from build123d import *

# Parameters (mm, degrees)
F0_R     = 1.5875
F1_DEPTH = 3.048


with BuildPart() as f1:
    # F0 (on Front) → F1 (new body)
    with BuildSketch(Plane.XZ):
        with BuildLine():
            Line((0, 112.7125), (0, 104.775))
            ThreePointArc((0, 104.775), (6.7351920908, 107.5648079092), (9.525, 114.3))
            Line((9.525, 114.3), (1.5875, 114.3))
            ThreePointArc((1.5875, 114.3), (1.1225320151, 113.1774679849), (0, 112.7125))
        make_face()
        with BuildLine():
            Line((-1.5875, 114.3), (-9.525, 114.3))
            ThreePointArc((-9.525, 114.3), (-6.7351920908, 107.5648079092), (0, 104.775))
            Line((0, 104.775), (0, 112.7125))
            ThreePointArc((0, 112.7125), (-1.1225320151, 113.1774679849), (-1.5875, 114.3))
        make_face()
        with BuildLine():
            ThreePointArc((9.525, 114.3), (0, 123.825), (-9.525, 114.3))
            Line((-9.525, 114.3), (-1.5875, 114.3))
            ThreePointArc((-1.5875, 114.3), (0, 115.8875), (1.5875, 114.3))
            Line((1.5875, 114.3), (9.525, 114.3))
        make_face()
        with BuildLine():
            Line((0, 104.775), (0, 79.375))
            ThreePointArc((0, 79.375), (10.0640474958, 75.7772380038), (15.5664511985, 66.6146784884))
            Line((15.5664511985, 66.6146784884), (9.5992867411, 114.3))
            Line((9.5992867411, 114.3), (9.525, 114.3))
            ThreePointArc((9.525, 114.3), (6.7351920908, 107.5648079092), (0, 104.775))
        make_face()
        with BuildLine():
            Line((-9.525, 114.3), (-15.7474569047, 65.5082893304))
            ThreePointArc((-15.7474569047, 65.5082893304), (-10.4912828548, 75.4142187767), (0, 79.375))
            Line((0, 79.375), (0, 104.775))
            ThreePointArc((0, 104.775), (-6.7351920908, 107.5648079092), (-9.525, 114.3))
        make_face()
        with Locations((-4.7625, 100.0252)):
            Circle(F0_R, mode=Mode.SUBTRACT)
        with BuildLine():
            ThreePointArc((-15.7942028036, 61.9003804205), (-10.644756084, 51.722700101), (0, 47.625))
            Line((0, 47.625), (0, 61.9125))
            ThreePointArc((0, 61.9125), (-1.5875, 63.5), (0, 65.0875))
            Line((0, 65.0875), (0, 79.375))
            ThreePointArc((0, 79.375), (-10.4912828548, 75.4142187767), (-15.7474569047, 65.5082893304))
            ThreePointArc((-15.7474569047, 65.5082893304), (-15.873667691, 63.7056672947), (-15.7942028036, 61.9003804205))
        make_face()
        with BuildLine():
            Line((0, 61.9125), (0, 47.625))
            ThreePointArc((0, 47.625), (10.644756084, 51.722700101), (15.7942028036, 61.9003804205))
            ThreePointArc((15.7942028036, 61.9003804205), (15.8547878338, 62.6991705884), (15.875, 63.5))
            ThreePointArc((15.875, 63.5), (15.7976744772, 65.0649620162), (15.5664511985, 66.6146784884))
            ThreePointArc((15.5664511985, 66.6146784884), (10.0640474958, 75.7772380038), (0, 79.375))
            Line((0, 79.375), (0, 65.0875))
            ThreePointArc((0, 65.0875), (1.1225320151, 64.6225320151), (1.5875, 63.5))
            ThreePointArc((1.5875, 63.5), (1.1225320151, 62.3774679849), (0, 61.9125))
        make_face()
        with BuildLine():
            Line((0, 47.625), (0, 9.525))
            ThreePointArc((0, 9.525), (6.7351920908, 6.7351920908), (9.525, 0))
            Line((9.525, 0), (36.5125, 0))
            ThreePointArc((36.5125, 0), (38.8373399243, 5.6126600757), (44.45, 7.9375))
            Line((44.45, 7.9375), (18.9329889534, 8.8488218231))
            ThreePointArc((18.9329889534, 8.8488218231), (13.22446249, 11.5691841219), (11.3070069952, 17.5950458731))
            Line((11.3070069952, 17.5950458731), (15.7942028036, 61.9003804205))
            ThreePointArc((15.7942028036, 61.9003804205), (10.644756084, 51.722700101), (0, 47.625))
        make_face()
        with BuildLine():
            ThreePointArc((-9.525, 0), (-6.7351920908, 6.7351920908), (0, 9.525))
            Line((0, 9.525), (0, 47.625))
            ThreePointArc((0, 47.625), (-10.644756084, 51.722700101), (-15.7942028036, 61.9003804205))
            Line((-15.7942028036, 61.9003804205), (-9.525, 0))
        make_face()
        with BuildLine():
            Line((0, 9.525), (0, 1.5875))
            ThreePointArc((0, 1.5875), (1.1225320151, 1.1225320151), (1.5875, 0))
            Line((1.5875, 0), (9.525, 0))
            ThreePointArc((9.525, 0), (6.7351920908, 6.7351920908), (0, 9.525))
        make_face()
        with BuildLine():
            ThreePointArc((-1.5875, 0), (-1.1225320151, 1.1225320151), (0, 1.5875))
            Line((0, 1.5875), (0, 9.525))
            ThreePointArc((0, 9.525), (-6.7351920908, 6.7351920908), (-9.525, 0))
            Line((-9.525, 0), (-1.5875, 0))
        make_face()
        with BuildLine():
            ThreePointArc((0, -1.5875), (-1.1225320151, -1.1225320151), (-1.5875, 0))
            Line((-1.5875, 0), (-9.525, 0))
            ThreePointArc((-9.525, 0), (-6.7351920908, -6.7351920908), (0, -9.525))
            Line((0, -9.525), (0, -1.5875))
        make_face()
        with BuildLine():
            Line((9.525, 0), (1.5875, 0))
            ThreePointArc((1.5875, 0), (1.1225320151, -1.1225320151), (0, -1.5875))
            Line((0, -1.5875), (0, -9.525))
            Line((0, -9.525), (0.6773435479, -9.500885786))
            ThreePointArc((0.6773435479, -9.500885786), (6.9705567315, -6.4912990883), (9.525, 0))
        make_face()
        with BuildLine():
            Line((36.5125, 0), (9.525, 0))
            ThreePointArc((9.525, 0), (6.9705567315, -6.4912990883), (0.6773435479, -9.500885786))
            Line((0.6773435479, -9.500885786), (44.45, -7.9425285691))
            Line((44.45, -7.9425285691), (44.45, -7.9375))
            ThreePointArc((44.45, -7.9375), (38.8373399243, -5.6126600757), (36.5125, 0))
        make_face()
        with BuildLine():
            Line((42.8625, 0), (36.5125, 0))
            ThreePointArc((36.5125, 0), (38.8373399243, -5.6126600757), (44.45, -7.9375))
            Line((44.45, -7.9375), (44.45, -1.5875))
            ThreePointArc((44.45, -1.5875), (43.3274679849, -1.1225320151), (42.8625, 0))
        make_face()
        with BuildLine():
            ThreePointArc((44.45, 7.9375), (38.8373399243, 5.6126600757), (36.5125, 0))
            Line((36.5125, 0), (42.8625, 0))
            ThreePointArc((42.8625, 0), (44.45, 1.5875), (46.0375, 0))
            ThreePointArc((46.0375, 0), (45.5725320151, -1.1225320151), (44.45, -1.5875))
            Line((44.45, -1.5875), (44.45, -7.9375))
            ThreePointArc((44.45, -7.9375), (50.0626600757, -5.6126600757), (52.3875, 0))
            ThreePointArc((52.3875, 0), (50.0626600757, 5.6126600757), (44.45, 7.9375))
        make_face()
    extrude(amount=F1_DEPTH)


solid = f1.part
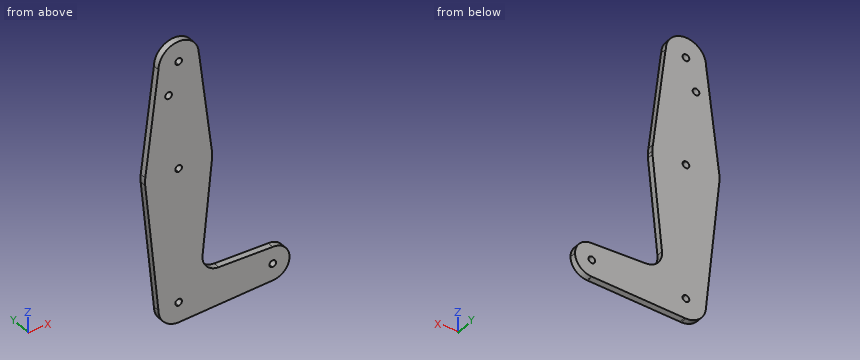
CAD build for the part. Positions are in the model's coordinates, mm. Round coordinates to 2 decimals unless told otherwise and drop trailing zeros. Write each loop counter-clockwise with the first axis right and the second up, starting at its lowest first coordinate (ties: lowest second). Pieces come first, ordered by that corner, then holes. Notation, with made-up numbers: (39.25, 21.5) -> (98.25, 21.5) arc R24 cw to (98.25, 43.5) -> close; hole circle Ø7 at (24, 86.25). An arc over 180 degrees is marked (long way). Answer as a JSON object with one key per item and string values.
(1) Band-saw the part on A-A, the plane y = -1. Count the separate pieces of the cut face and the enclosed holes in it, then the cut area to 3 significant figures.
Reported:
{"separate pieces": "1", "enclosed holes": "5", "area": "3,890 mm^2"}
(2) Probe probe 1 along X at (y, z) = (-0.55, -0.5); probe 2 along X at (y, z) = (-2.85, 104); probe 3 along X at (y, z) = (-2.9, 32). List the from-to ranges inside material, lowest first. Write a range as [from, to].
Reported:
{"probe 1": "x = [-9.51, -1.51], [1.51, 42.94], [45.96, 52.37]", "probe 2": "x = [-10.84, 10.89]", "probe 3": "x = [-12.77, 12.77]"}
(3) Band-saw the part on B-B, the plane z = 49. List the corners of the cut face in (x, y).
Reported:
{"outline": "(-14.49, -3.05) -> (14.49, -3.05) -> (14.49, 0) -> (-14.49, 0) -> close"}
(4) Pin check, flat tips, straight feed: P1, Ø1, axis at x = 3.5, y = -2, coming from the -Z side; P2, Ø1.5, axis at x = 27.5, y = -2, coming from the -Z side. Stop position of each tip, or through.
Reported:
{"P1": "stops at z = -9.42", "P2": "stops at z = -8.57"}
(5) Band-saw the part on C-C, the plane x = 47.5. List the corners of the cut face in (y, z), then the cut area to 3 significant figures.
Reported:
{"outline": "(-3.05, -7.33) -> (0, -7.33) -> (0, 7.33) -> (-3.05, 7.33) -> close", "area": "44.7 mm^2"}
